For this review, use the dimensioned drawing (mm, ordinates from the lowest corner) and the shaded views. Round coordinates to 2 decimals unless told otherwise and drop trailing zeros. Write each loop counter-clockwise with the first axis right and the second up, starting at its lowest first coordinate (ties: lowest second). Pieces come first, ordered by that corner, then holes.
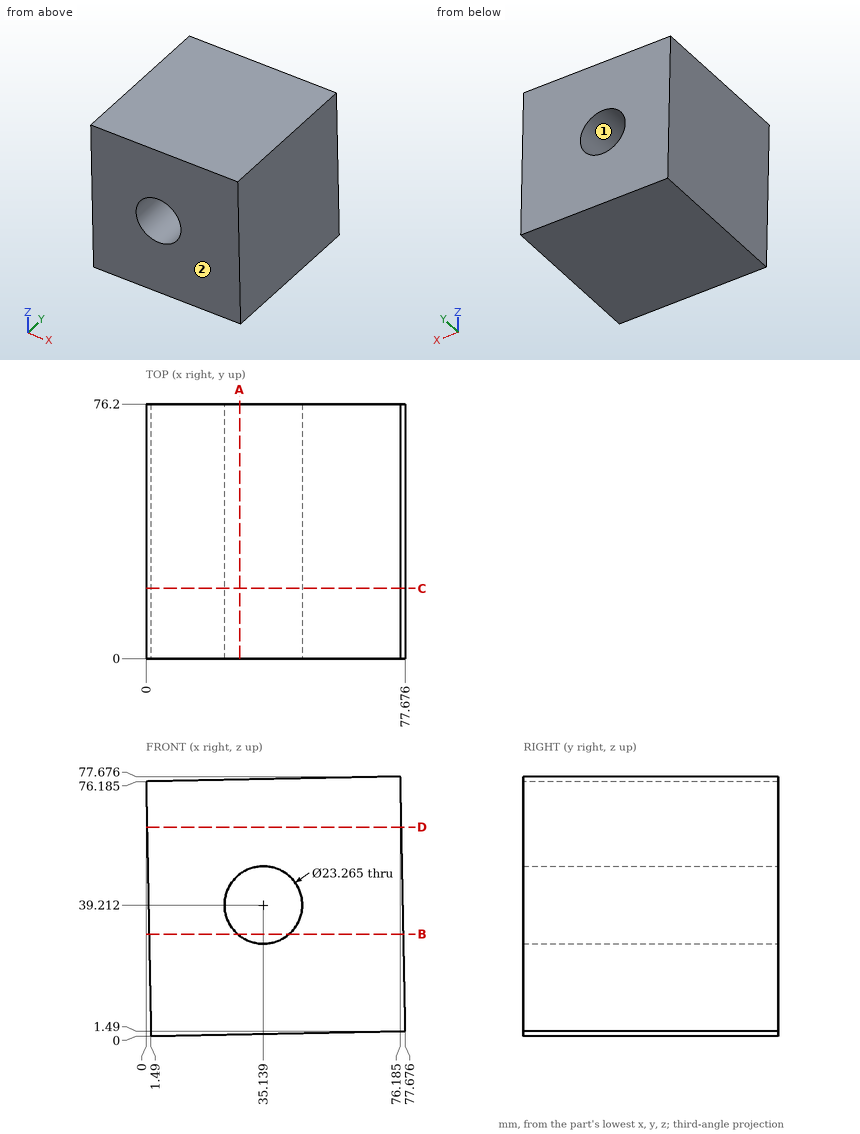
(1) For line 1 along X through (y, z) = (6, 40.5); line 2 along X through (y, z) = (30, 34) (1 decimal); line 3 along Z through (x, y) = (30, 52.5) (1 decimal), list the stretches that pass through material, from the lowest coordinate up.
Geometry check:
line 1: x = 0.7 to 23.58, 46.7 to 76.91
line 2: x = 0.8 to 24.7, 45.5 to 77
line 3: z = 0.6 to 28.8, 49.6 to 76.8
(2) We need section D-D, the plane z = 62.5. Give the boundary of the cut face in (x, y), and give its area (3 significant figures).
Geometry check:
outline: (0.27, 0) - (76.48, 0) - (76.48, 76.2) - (0.27, 76.2) - close
area: 5,810 mm2
(3) We need section A-A, the plane x = 28. Give the boundary of the cut face in (y, z).
Geometry check:
outline: (0, 0.52) - (76.2, 0.52) - (76.2, 30.03) - (0, 30.03) - close; (0, 48.4) - (76.2, 48.4) - (76.2, 76.73) - (0, 76.73) - close
(4) We need section B-B, the plane z = 30.5. Give the boundary of the cut face in (x, y).
Geometry check:
outline: (0.89, 0) - (27.43, 0) - (27.43, 76.2) - (0.89, 76.2) - close; (42.85, 0) - (77.11, 0) - (77.11, 76.2) - (42.85, 76.2) - close
(5) We need section C-C, the plane y = 21. Give the boundary of the cut face in (x, z) (1 decimal), and give its area (3 significant figures).
Geometry check:
outline: (0, 76.2) - (1.5, 0) - (77.7, 1.5) - (76.2, 77.7) - close; hole circle Ø23.3 at (35.1, 39.2)
area: 5,380 mm2
(6) For pin 1 Ø1 at (y, z) = (49, 68.5) entering from +X (1 decimal); pin 2 Ø8 at (y, z) = (49, 67) entering from +X; pin 3 Ø5 at (y, z) = (61.5, 55.5) entering from -X, all flat-tipped, find the tip position at first contact; note any pin that passes through.
Geometry check:
pin 1: stops at x = 76.4
pin 2: stops at x = 76.47
pin 3: stops at x = 0.36
(7) Mouldability with a two-part tool opening along Z and no side actions: class the marked faces 1 and 2 as pulls with the +Z half, pulls with the -Z half, needs draft (parallel to the pull), parting line crosses it, or undercut.
Geometry check:
face 1: undercut
face 2: needs draft
